Part model, mm, in its own coordinate system. A direction names the side the tool comes from. Round coordinates to 2 decimals unless told otherwise and drop trailing zeros. Write each loop counter-clockwise with the first axis right and the second up, starting at its lowest first coordinate (ties: lowest second). Pieces come first, ordered by that corner, then holes.
```python
from build123d import *

# Parameters (mm, degrees)
ESQUISSE2_W = 2
ESQUISSE2_H = 12


with BuildPart() as part:
    # Esquisse2 → Révolution2 (revolve)
    with BuildSketch(Plane.XY, mode=Mode.PRIVATE) as r_volution2_sk:
        Polygon((2, 32.533333333), (0, 32.533333333), (0, 1.533333333), (12.2, 1.533333333), (12.2, 32.533333333), align=None)
        with Locations((1, 38.533333333)):
            Rectangle(ESQUISSE2_W, ESQUISSE2_H)
        Polygon((12.2, 1.533333333), (0, 1.533333333), (0, -19.466666667), (12.5, -19.466666667), (12.5, 1.533333333), align=None)
    revolve(r_volution2_sk.sketch.rotate(Axis((0, 32.533333333, 0), (0, -1, 0)), 180), axis=Axis((0, 32.533333333, 0), (0, -1, 0)))


solid = part.part
```
Q1. Drop flat-ended pins along their axis: pin 1 (12 mm diameter, centred on x = 6, y = 26.5, fed in from +Z); pin 2 (3 mm diameter, centred on y = 25.5, z = 7, fed in from -X); pin 3 (10 mm diameter, centred on y = 15, z = -5, fed in from +X). Give the stop position or say it passes through.
Values follow:
pin 1: stops at z = 12.2
pin 2: stops at x = -10.89
pin 3: stops at x = 12.2
Q2. Which spindle directions (+Z, -Z, +X, -X, +Y, -Y) get a long thin tool onto all of the face, cutting with end or side? Do faces 1 (the cylindrical face through (0, 39, 2)), 2 (the flat face through (0, -19.467, 0)). Say none if no direction does.
Values follow:
face 1: +Y
face 2: +Z, -Z, +X, -X, -Y
Q3. Wall check: L1, parallel to Y at x = -2.5, z = 9.5; L2, parallel to Z at x = -0.25, y = -8; L3, parallel to Z at x = -10, y = -17. Give the ranges that are in metal, low to high.
Values follow:
L1: y = -19.47 to 32.53
L2: z = -12.5 to 12.5
L3: z = -7.5 to 7.5
Q4. Cut at C-C on y = -4. Write the cut outline in (x, z).
Values follow:
outline: circle Ø25 at (0, 0)
Q5. Cut at A-A on z = 0. Write the cut outline in (x, y).
Values follow:
outline: (-12.5, -19.47) - (12.5, -19.47) - (12.5, 1.53) - (12.2, 1.53) - (12.2, 32.53) - (2, 32.53) - (2, 44.53) - (-2, 44.53) - (-2, 32.53) - (-12.2, 32.53) - (-12.2, 1.53) - (-12.5, 1.53) - close
Q6. Cut at D-D on z = 9. Write the cut outline in (x, y), plus the area to 3 significant figures.
Values follow:
outline: (-8.67, -19.47) - (8.67, -19.47) - (8.67, 1.53) - (8.24, 1.53) - (8.24, 32.53) - (-8.24, 32.53) - (-8.24, 1.53) - (-8.67, 1.53) - close
area: 875 mm2
Q7. Cut at B-B on x = 0. Write the cut outline in (y, z).
Values follow:
outline: (-19.47, -12.5) - (1.53, -12.5) - (1.53, -12.2) - (32.53, -12.2) - (32.53, -2) - (44.53, -2) - (44.53, 2) - (32.53, 2) - (32.53, 12.2) - (1.53, 12.2) - (1.53, 12.5) - (-19.47, 12.5) - close
